Input: part model. Units: mm. Frame: model coordinates. Face numbers are marked on the shaded views. A direction names the side the tool comes from. Coordinates: 2 decimals unless noted, no trailing zeros. Order: outer loops, then holes, each group sorted by start corner. A loop starts at its lowest first (then second) coordinate and runs counter-clockwise, first axis right, second up. Notation, with made-up numbers: (-18, 24) -> (-13, 24) arc R30 ccw to (-13, 59) -> close; hole circle Ø4 at (34, -19.75). An arc over 180 degrees is marked (long way). Use one line per item in the form item = value. Start each with the question number.
1) Section query A-A on x = -9. Output: boundary loops of the cut face in (y, z), then the cut area to 3 significant figures.
2) Pin query (flat end, axial travel): pin 1 (2.5 mm diameter, centred on x = -17, y = 2.5, fed in from +Z); pin 2 (1.2 mm diameter, centred on x = -18, z = 12.5, fed in from -Y); pin 3 (5 mm diameter, centred on x = -53, z = 7.5, fed in from +Y); pin 4 (1.5 mm diameter, centred on x = 11.5, z = 10.5, fed in from -Y). Return the tip coordinate at first contact, or that it passes through.
3) Access query for the marked faces 1, 2 and 3. Directions: +Z, -Z, +X, -X, +Y, -Y. A direction counts if a zero-diameter tool reaches every point of the face in a straight line with its end or side. Return the directions, or none.
4) Draft query along X for the marked faces 4, 5 and 6. Return one class per face: pulls with the +X half, pulls with the -X half, needs draft (parallel to the pull), parting line crosses it, or undercut.
5) Section query B-B on z = 15.25. Count the separate pieces of the cut face and the enclosed holes in it, then the cut area to 3 significant figures.
6) Ray query, line 1 along Y through (x, z) = (-49.5, 5.25); line 2 along Y through (x, z) = (-20, 11); line 3 along X through (y, z) = (-2.75, 2). Return the intervals inside material, ascending.
7) Section query D-D on y = 10. Output: boundary loops of the cut face in (x, z), then the cut area to 3 significant figures.
from build123d import *

# Parameters (mm, degrees)
SKETCH_1_W          = 35
SKETCH_1_H          = 17
EXTRUDE_1_DEPTH     = 4
SKETCH_2_W          = 24
SKETCH_2_H          = 13
CUT_EXTRUDE_1_DEPTH = 6
EXTRUDE_2_DEPTH     = 5
SKETCH_5_W          = 4
SKETCH_5_H          = 4
SKETCH_5_R          = 1.15
EXTRUDE_3_DEPTH     = 15
SKETCH_6_R          = 1.15
CUT_EXTRUDE_2_DEPTH = 15
EXTRUDE_5_DEPTH     = 2
EXTRUDE_6_DEPTH     = 4
CUT_EXTRUDE_3_DEPTH = 3
SKETCH_11_R         = 1.25
CUT_EXTRUDE_4_DEPTH = 13.4


with BuildPart() as part:
    # 草圖1 → 填料-伸長1 (new body)
    with BuildSketch(Plane.XY):
        with Locations((-3.721052632, 2.8)):
            Rectangle(SKETCH_1_W, SKETCH_1_H)
    extrude(amount=EXTRUDE_1_DEPTH)

    # 草圖2 → 除料-伸長1 (cut)
    with BuildSketch(Plane.XY):
        with Locations((-3.221052632, 2.8)):
            Rectangle(SKETCH_2_W, SKETCH_2_H)
    extrude(amount=CUT_EXTRUDE_1_DEPTH, mode=Mode.SUBTRACT)

    # 草圖3 → 填料-伸長2 (add)
    with BuildSketch(Plane(origin=(13.778947368, 0, 0), x_dir=(0, 0, -1), z_dir=(1, 0, 0))):
        Polygon((-4, 7.802538439), (-4, 11.3), (-19, 11.3), (-19, -5.694923122), (-4, -5.694923122), (-4, -2.197461561), (-9, -2.197461561), (-9, 7.802538439), align=None)
    extrude(amount=-EXTRUDE_2_DEPTH)

    # 草圖5 → 填料-伸長3 (add)
    with BuildSketch(Plane.XY.offset(4)):
        with Locations((-17.221052632, 2.8)):
            Rectangle(SKETCH_5_W, SKETCH_5_H)
        with Locations((-17.221052632, 2.8)):
            Circle(SKETCH_5_R, mode=Mode.SUBTRACT)
    extrude(amount=EXTRUDE_3_DEPTH)

    # 草圖6 → 除料-伸長2 (cut)
    with BuildSketch(Plane.XY.offset(19)):
        with Locations((11.278947368, 2.802538439)):
            Circle(SKETCH_6_R)
    extrude(amount=-CUT_EXTRUDE_2_DEPTH, mode=Mode.SUBTRACT)

    # 草圖7 → 填料-伸長5 (add)
    with BuildSketch(Plane.ZY.offset(21.221052632)):
        Polygon((4, 4.8), (4, 0.796544916), (19, 0.8), (19, 4.8), align=None)
    extrude(amount=-EXTRUDE_5_DEPTH)

    # 草圖9 → 填料-伸長6 (add)
    with BuildSketch(Plane(origin=(0, 0.8, 0), x_dir=(-1, 0, 0), z_dir=(0, -1, 0))):
        with BuildLine():
            Line((21.221052632, -1.209797885), (21.221052632, -16.209797885))
            Line((21.221052632, -16.209797885), (61.221052632, -16.209797885))
            ThreePointArc((61.221052632, -16.209797885), (68.721052632, -8.709797885), (61.221052632, -1.209797885))
            Line((61.221052632, -1.209797885), (21.221052632, -1.209797885))
        make_face()
    extrude(amount=-EXTRUDE_6_DEPTH)

    # 草圖10 → 除料-伸長3 (cut)
    with BuildSketch(Plane(origin=(0, 4.8, 0), x_dir=(1, 0, 0), z_dir=(0, 1, 0))):
        with BuildLine():
            Line((-45.267861932, -3.783815128), (-62.253576218, -6.739404782))
            ThreePointArc((-62.253576218, -6.739404782), (-63.910719075, -8.709797885), (-62.253576218, -10.680190988))
            Line((-62.253576218, -10.680190988), (-45.267861932, -13.635780642))
            ThreePointArc((-45.267861932, -13.635780642), (-44.410719075, -13.709797885), (-43.553576218, -13.635780642))
            Line((-43.553576218, -13.635780642), (-26.567861932, -10.680190988))
            ThreePointArc((-26.567861932, -10.680190988), (-24.910719075, -8.709797885), (-26.567861932, -6.739404782))
            Line((-26.567861932, -6.739404782), (-43.553576218, -3.783815128))
            ThreePointArc((-43.553576218, -3.783815128), (-44.410719075, -3.709797885), (-45.267861932, -3.783815128))
        make_face()
    extrude(amount=-CUT_EXTRUDE_3_DEPTH, mode=Mode.SUBTRACT)

    # 草圖11 → 除料-伸長4 (cut)
    with BuildSketch(Plane(origin=(0, 4.8, 0), x_dir=(1, 0, 0), z_dir=(0, 1, 0))):
        with Locations((-44.410719075, -8.709797885)):
            Circle(SKETCH_11_R)
    extrude(amount=-CUT_EXTRUDE_4_DEPTH, mode=Mode.SUBTRACT)


solid = part.part
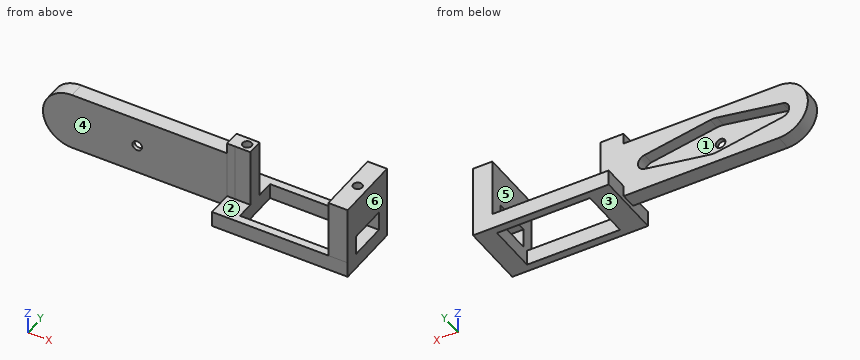
Answers below:
q1.outline = (-5.7, 0) -> (-3.7, 0) -> (-3.7, 4) -> (-5.7, 4) -> close; (9.3, 0) -> (11.3, 0) -> (11.3, 4) -> (9.3, 4) -> close
q1.area = 16.0 mm^2
q2.pin_1 = 19
q2.pin_2 = 0.8
q2.pin_3 = 4.8
q2.pin_4 = -5.69
q3.face_1 = +Y
q3.face_2 = +Z, -X, -Y
q3.face_3 = -Z, +X, -X, +Y, -Y
q4.face_4 = needs draft
q4.face_5 = undercut
q4.face_6 = pulls with the +X half
q5.separate_pieces = 2
q5.enclosed_holes = 2
q5.area = 275 mm^2
q6.line_1 = 0.8 to 1.8
q6.line_2 = 0.8 to 4.8
q6.line_3 = -21.22 to -15.22, 8.78 to 13.78
q7.outline = (-21.22, 0) -> (13.78, 0) -> (13.78, 19) -> (8.78, 19) -> (8.78, 4) -> (-21.22, 4) -> close
q7.area = 215 mm^2
